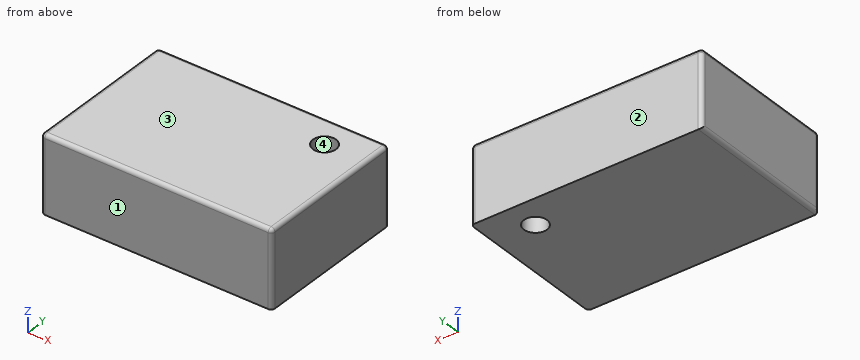
```python
from build123d import *

# Parameters (mm, degrees)
F0_W     = 300
F0_H     = 200
F0_R     = 15
F1_DEPTH = 100
F2_R     = 5


with BuildPart() as f1:
    # F0 (on Top) → F1 (new body)
    with BuildSketch(Plane.XY):
        with Locations((1.263371, 9.330785)):
            Rectangle(F0_W, F0_H)
        with Locations((97.774066, 69.591478)):
            Circle(F0_R, mode=Mode.SUBTRACT)
    extrude(amount=F1_DEPTH)

    # F2
    f2_edges = [f1.edges().sort_by_distance(p)[0] for p in [
        (-148.736629, 109.330785, 50),
        (151.263371, 109.330785, 50),
        (1.263371, 109.330785, 100),
        (151.263371, 9.330785, 100),
        (-148.736629, 9.330785, 100),
        (1.263371, -90.669215, 100),
        (-148.736629, -90.669215, 50),
        (-148.736629, 9.330785, 0),
        (151.263371, -90.669215, 50),
    ]]
    fillet(f2_edges, radius=F2_R)


solid = f1.part
```
Design review of the part built by this model. Coordinates are the model's own, in mm. Face numbers are marked on the shaded views. Give positions to 0.01 mm unless a question says otherwise; leave off trailing zeros. Loops run counter-clockwise (first coordinate to the right, second up) from the corner with the lowest first, then second, coordinate; pieces in that order, holes last. Notation, with made-up numbers: M 3.5,-26 L 22.5,-26 A24 ccw 22.5,-1 Z; hole C 48,17 d8. An arc over 180 degrees is marked long. Return JSON: item names as keys, results as strings. Group by question number.
Item 1: For probe 1 along X at (y, z) = (82.5, 72); probe 2 along X at (y, z) = (58, 32), list the stretches that pass through material, from the lowest coordinate up.
Item 2: We need section A-A (y = 80.5). Give the boundary of the cut face in (x, z).
Item 3: Mouldability with a two-part tool opening along Y and no side actions: class the marked faces 1, 2, 3 and 4 as released by +Y, released by -Y, zero draft, split by the parting line, or undercut.
Output:
{
 "1": {"probe 1": "x = -148.74 to 90.13, 105.41 to 151.26", "probe 2": "x = -148.74 to 88.25, 107.29 to 151.26"},
 "2": {"outline": "M -148.74,5 A5 ccw -143.74,0 L 87.48,0 L 87.48,100 L -143.74,100 A5 ccw -148.74,95 Z; M 108.07,0 L 151.26,0 L 151.26,95 A5 ccw 146.26,100 L 108.07,100 Z"},
 "3": {"face 1": "released by -Y", "face 2": "released by +Y", "face 3": "zero draft", "face 4": "undercut"}
}
